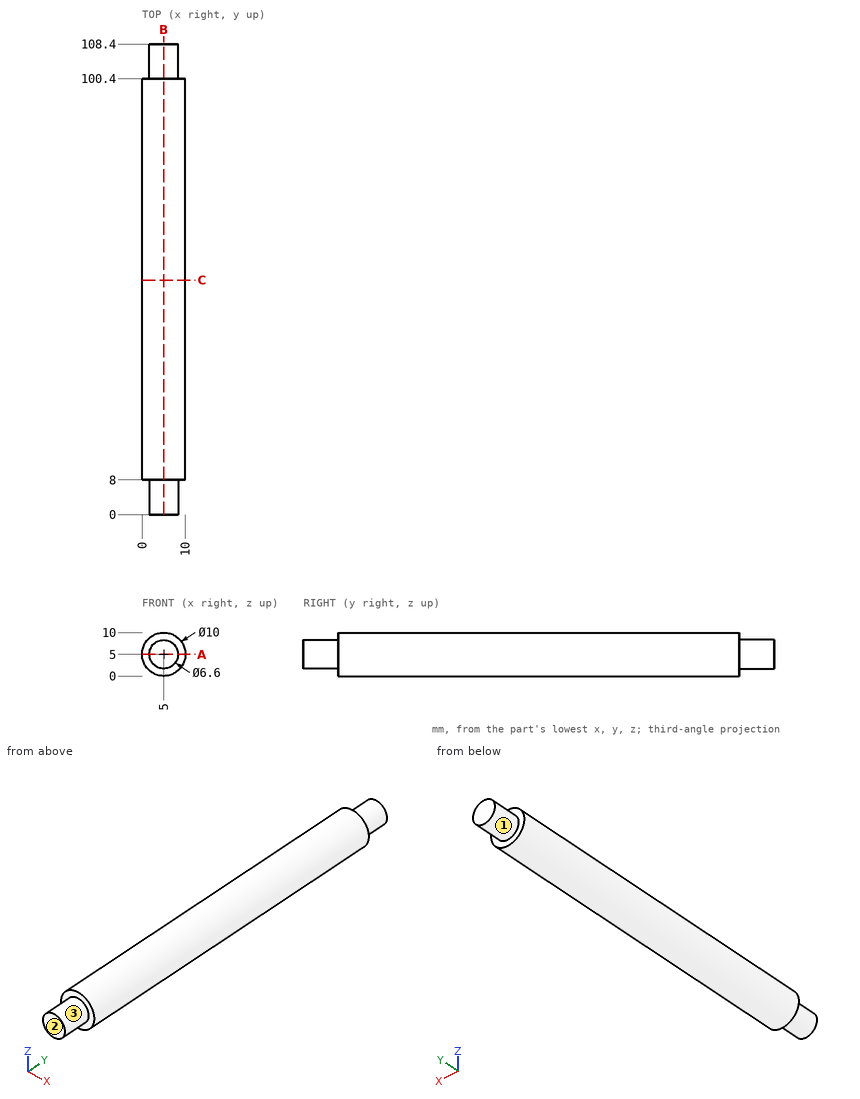
For this review, use the dimensioned drawing (mm, ordinates from the lowest corner) and the shaded views. A direction names the side the tool comes from. Round coordinates to 2 decimals unless told otherwise and drop trailing zeros. Write each loop counter-clockwise with the first axis right and the second up, starting at its lowest first coordinate (ties: lowest second). Pieces come first, ordered by that corner, then holes. Notation, with made-up numbers: (44.5, -15) - (65.5, -15) arc R16 cw to (65.5, 13) - close; hole circle Ø1 at (9.25, -40). An arc over 180 degrees is marked (long way). Answer as CSV lines item,"result". Start each with the question number.
(1) We need section C-C on y = 54. State the section outline as (x, z) points, plus the area to 3 significant figures.
(2) For pin 1 Ø1.5 at (x, y) = (3.5, 15) entering from +Z; pin 2 Ø4 at (x, y) = (8.5, 19.5) entering from -Z; pin 3 Ø3 at (y, z) = (38, 9) entering from -X, all flat-tipped, find the tip position at first contact; note any pin that passes through.
(3) We need section B-B on x = 5. State the section outline as (y, z) points, plus the area to 3 significant figures.
(4) We need section A-A on z = 5. State the section outline as (x, y) points.
(5) To check wall thickness, follow line 1 (Y direction, x = 7.75, z = 2.5); line 2 (Z direction, x = 8.75, y = 78); line 3 (X direction, y = 32.5, z = 4.75). State the ranges of each line that lie inside material, in increasing order.
(6) For the marked faces 1, 2 and 3, list the 3-axis set-ups (+Z, -Z, +X, -X, +Y, -Y) from which the entire face can be reached by the end or side of a thin tool; tool diameter is ignored.
Worked answers:
1,outline,"circle Ø10 at (5, 5)"
1,area,"78.5 mm²"
2,pin 1,"z = 9.94"
2,pin 2,"z = 0.23"
2,pin 3,"x = 0.67"
3,outline,"(0, 1.7) - (8, 1.7) - (8, 0) - (100.4, 0) - (100.4, 1.7) - (108.4, 1.7) - (108.4, 8.3) - (100.4, 8.3) - (100.4, 10) - (8, 10) - (8, 8.3) - (0, 8.3) - close"
3,area,"1,030 mm²"
4,outline,"(0, 8) - (1.7, 8) - (1.7, 0) - (8.3, 0) - (8.3, 8) - (10, 8) - (10, 100.4) - (8.3, 100.4) - (8.3, 108.4) - (1.7, 108.4) - (1.7, 100.4) - (0, 100.4) - close"
5,line 1,"8 to 100.4"
5,line 2,"1.69 to 8.31"
5,line 3,"0.01 to 9.99"
6,face 1,"+Y"
6,face 2,"+Z, -Z, +X, -X, -Y"
6,face 3,"-Y"
